```python
from build123d import *

# Parameters (mm, degrees)
BOSS_EXTRUDE1_DEPTH = 18
SKETCH2_R           = 12.45
SKETCH2_R_2         = 9.45
BOSS_EXTRUDE2_DEPTH = 10
SKETCH3_R           = 12.45
BOSS_EXTRUDE3_DEPTH = 2
CUT_EXTRUDE1_REACH  = 30.085
SKETCH4_R           = 1.45
CUT_EXTRUDE2_START  = -8
CUT_EXTRUDE2_DEPTH  = 3
CUT_EXTRUDE3_REACH  = 35.076
BOSS_EXTRUDE4_START = -5
BOSS_EXTRUDE4_DEPTH = 5
SKETCH8_R           = 1.5
CUT_EXTRUDE4_DEPTH  = 30.783714089


with BuildPart() as part:
    # Sketch1 → Boss-Extrude1 (new body)
    with BuildSketch(Plane(origin=(0, 0, 0), x_dir=(1, 0, 0), z_dir=(0, 1, 0))):
        with BuildLine():
            Line((-5.149418526, 2.325078245), (-5.149418526, -2.325078245))
            ThreePointArc((-5.149418526, -2.325078245), (5.65, 0), (-5.149418526, 2.325078245))
        make_face()
        with BuildLine():
            Line((-2.124418526, 1.541904967), (-2.124418526, -1.541904967))
            ThreePointArc((-2.124418526, -1.541904967), (2.625, 0), (-2.124418526, 1.541904967))
        make_face(mode=Mode.SUBTRACT)
    extrude(amount=BOSS_EXTRUDE1_DEPTH)



with BuildPart() as body_2:
    # Sketch2 → Boss-Extrude2 (new body)
    with BuildSketch(Plane.XZ):
        with Locations(Location((0, 0, 0), (0, 0, 270))):
            Circle(SKETCH2_R)
        with Locations(Location((0, 0, 0), (0, 0, 270))):
            Circle(SKETCH2_R_2, mode=Mode.SUBTRACT)
    extrude(amount=BOSS_EXTRUDE2_DEPTH)


with BuildPart() as part_1:
    add(part.part)

    add(body_2.part)  # Boss-Extrude3 merges body 2
    # Sketch3 → Boss-Extrude3 (add)
    with BuildSketch(Plane.XZ):
        with Locations(Location((0, 0, 0), (0, 0, 270))):
            Circle(SKETCH3_R)
    extrude(amount=BOSS_EXTRUDE3_DEPTH)

    # Sketch4 → Cut-Extrude1 (cut, up to next)
    with BuildSketch(Plane.ZY.offset(5.149418526), mode=Mode.PRIVATE) as cut_extrude1_sk1:
        with Locations((0, 14)):
            Circle(SKETCH4_R)
    cut_extrude1_tool1 = extrude(cut_extrude1_sk1.sketch, amount=-CUT_EXTRUDE1_REACH, mode=Mode.PRIVATE) & part_1.part
    # Sketch4 → Cut-Extrude1 (cut, up to next)
    with BuildSketch(Plane.ZY.offset(5.149418526), mode=Mode.PRIVATE) as cut_extrude1_sk2:
        with Locations((0, 4)):
            Circle(SKETCH4_R)
    cut_extrude1_tool2 = extrude(cut_extrude1_sk2.sketch, amount=-CUT_EXTRUDE1_REACH, mode=Mode.PRIVATE) & part_1.part
    add(cut_extrude1_tool1.solids().sort_by_distance((-5.149419, 14, 0))[0], mode=Mode.SUBTRACT)
    add(cut_extrude1_tool2.solids().sort_by_distance((-5.149419, 4, 0))[0], mode=Mode.SUBTRACT)

    # Sketch5 → Cut-Extrude2 (cut)
    with BuildSketch(Plane.XZ.offset(10).offset(CUT_EXTRUDE2_START)):
        with BuildLine():
            Line((-8.961166219, 3), (-12.083149424, 3))
            ThreePointArc((-12.083149424, 3), (0, 12.45), (12.083149424, 3))
            Line((12.083149424, 3), (8.961166219, 3))
            ThreePointArc((8.961166219, 3), (0, 9.45), (-8.961166219, 3))
        make_face()
        with BuildLine():
            Line((-8.961166219, -3), (-12.083149424, -3))
            ThreePointArc((-12.083149424, -3), (0, -12.45), (12.083149424, -3))
            Line((12.083149424, -3), (8.961166219, -3))
            ThreePointArc((8.961166219, -3), (0, -9.45), (-8.961166219, -3))
        make_face()
    extrude(amount=CUT_EXTRUDE2_DEPTH, mode=Mode.SUBTRACT)

    # Sketch6 → Cut-Extrude3 (cut, up to next)
    with BuildSketch(Plane.XZ.offset(10), mode=Mode.PRIVATE) as cut_extrude3_sk1:
        with BuildLine():
            Line((0.75, 9.420191081), (0.75, 12.427389106))
            ThreePointArc((0.75, 12.427389106), (0, 12.45), (-0.75, 12.427389106))
            Line((-0.75, 12.427389106), (-0.75, 9.420191081))
            ThreePointArc((-0.75, 9.420191081), (0, 9.45), (0.75, 9.420191081))
        make_face()
    cut_extrude3_tool1 = extrude(cut_extrude3_sk1.sketch, amount=-CUT_EXTRUDE3_REACH, mode=Mode.PRIVATE) & part_1.part
    # Sketch6 → Cut-Extrude3 (cut, up to next)
    with BuildSketch(Plane.XZ.offset(10), mode=Mode.PRIVATE) as cut_extrude3_sk2:
        with BuildLine():
            Line((0.75, -9.420191081), (0.75, -12.427389106))
            ThreePointArc((0.75, -12.427389106), (0, -12.45), (-0.75, -12.427389106))
            Line((-0.75, -12.427389106), (-0.75, -9.420191081))
            ThreePointArc((-0.75, -9.420191081), (0, -9.45), (0.75, -9.420191081))
        make_face()
    cut_extrude3_tool2 = extrude(cut_extrude3_sk2.sketch, amount=-CUT_EXTRUDE3_REACH, mode=Mode.PRIVATE) & part_1.part
    add(cut_extrude3_tool1.solids().sort_by_distance((0, -10, 10.941262))[0], mode=Mode.SUBTRACT)
    add(cut_extrude3_tool2.solids().sort_by_distance((0, -10, -10.941262))[0], mode=Mode.SUBTRACT)

    # Sketch7 → Boss-Extrude4 (add)
    with BuildSketch(Plane.XZ.offset(10).offset(BOSS_EXTRUDE4_START)):
        with BuildLine():
            ThreePointArc((-2.25, 12.244998979), (-1.502769623, 12.35897178), (-0.75, 12.427389106))
            Line((-0.75, 12.427389106), (-0.75, 18.627389106))
            Line((-0.75, 18.627389106), (-2.25, 18.627389106))
            Line((-2.25, 18.627389106), (-2.25, 12.244998979))
        make_face()
        with BuildLine():
            Line((2.25, 12.244998979), (2.25, 18.627389106))
            Line((2.25, 18.627389106), (0.75, 18.627389106))
            Line((0.75, 18.627389106), (0.75, 12.427389106))
            ThreePointArc((0.75, 12.427389106), (1.502769623, 12.35897178), (2.25, 12.244998979))
        make_face()
        with BuildLine():
            ThreePointArc((-0.75, -12.427389106), (-1.502769623, -12.35897178), (-2.25, -12.244998979))
            Line((-2.25, -12.244998979), (-2.25, -18.627389106))
            Line((-2.25, -18.627389106), (-0.75, -18.627389106))
            Line((-0.75, -18.627389106), (-0.75, -12.427389106))
        make_face()
        with BuildLine():
            Line((2.25, -18.627389106), (2.25, -12.244998979))
            ThreePointArc((2.25, -12.244998979), (1.502769623, -12.35897178), (0.75, -12.427389106))
            Line((0.75, -12.427389106), (0.75, -18.627389106))
            Line((0.75, -18.627389106), (2.25, -18.627389106))
        make_face()
    extrude(amount=BOSS_EXTRUDE4_DEPTH)

    # Sketch8 → Cut-Extrude4 (cut, through all)
    with BuildSketch(Plane.ZY.offset(2.25)):
        with Locations(Location((-15.436194043, -7.5, 0), (0, 0, 180))):
            Circle(SKETCH8_R)
        with Locations((15.436194043, -7.5)):
            Circle(SKETCH8_R)
    extrude(amount=-CUT_EXTRUDE4_DEPTH, mode=Mode.SUBTRACT)


solid = part_1.part
```
Part model, mm, in its own coordinate system. A direction names the side the tool comes from. Give positions to 0.01 mm unless a question says otherwise; leave off trailing zeros. Order: outer loops, then holes, each group sorted by start corner. A loop starts at its lowest first (then second) coordinate and runs counter-clockwise, first axis right, second up. Notation, with made-up numbers: M 14,74 L 39,74 A22 ccw 39,101 Z; hole C 37,-38 d6. An arc over 180 degrees is marked long. Use a Markdown table: item, result. Add a question column.
(1) Mould opens along Z. For faces 1 (the face through (1, -7, -18.627)), 2 (the face through (1.49, -6.925, -16.822)), 3 (the face through (-9.448, -6.833, 0.197)), 4 (the face through (2.25, -5.8, -15.5)) say: +Z half, -Z half, draft (parallel to the pull), parting line (faces both ways), or undercut.
(2) Saw through at A-A, the plane z = 0. Give the cut face in (x, y) (3 decimals).
(3) 3-axis set-ups, long thin cutter, end or side, ignore diameter. For faces 5 (the face through (2.25, -5.8, 15.4)), 6 (the face through (-2.124, 9, 0)), 7 (the face through (11, -3, -3)): which of +Z, -Z, +X, -X, +Y, -Y reach the whole face in a straight line?
(4) Saw through at B-B, the plane y = -7.5. Give the number of separate pieces and of enclosed holes in the cut face, and give its area (3 significant figures).
(5) Saw through at C-C, the plane x = -1.5. Give the cut face in (y, z).
(6) Saw through at D-D, the plane x = 7. Give the cut face in (y, z), and give its area (3 significant figures).
(7) Probe line 1 along Y through (x, z) = (-3.65, 0); line 2 along Y through (x, z) = (-9.25, 5.5); line 3 along Y through (x, z) = (-7, 4.5). List the from-to ranges inside material, lowest first. Write a range as [from, to].
(8) Drop flat-ended pins along their axis: P1, Ø10, axis at x = 8.5, y = -1, coming from the -Z side; P2, Ø8, axis at x = 8.5, z = -7, coming from the +Y side; P3, Ø2.5, axis at y = 11.5, z = -0.5, coming from the +X side. Give the stop position or say it passes through.
Answer key:
| question | item | result |
|---|---|---|
| 1 | face 1 | -Z half |
| 1 | face 2 | undercut |
| 1 | face 3 | undercut |
| 1 | face 4 | draft |
| 2 | outline | M -12.45,-10 L -9.45,-10 L -9.45,-2 L 9.45,-2 L 9.45,-10 L 12.45,-10 L 12.45,0 L 5.65,0 L 5.65,18 L 2.625,18 L 2.625,0 L -2.124,0 L -2.124,2.55 L -5.149,2.55 L -5.149,0 L -12.45,0 Z; M -5.149,5.45 L -2.124,5.45 L -2.124,12.55 L -5.149,12.55 Z; M -5.149,15.45 L -2.124,15.45 L -2.124,18 L -5.149,18 Z |
| 3 | face 5 | +Z, +X, +Y, -Y |
| 3 | face 6 | +Y |
| 3 | face 7 | -Z, +X, -X |
| 4 | separate pieces | 6 |
| 4 | enclosed holes | 0 |
| 4 | area | 217 mm^2 |
| 5 | outline | M -10,-18.63 L -5,-18.63 L -5,-9.33 L -10,-9.33 Z; M -10,9.33 L -5,9.33 L -5,18.63 L -10,18.63 Z; M -2,-12.36 L 0,-12.36 L 0,-5.45 L 18,-5.45 L 18,-2.15 L 0,-2.15 L 0,2.15 L 18,2.15 L 18,5.45 L 0,5.45 L 0,12.36 L -2,12.36 Z; hole C -7.5,-15.44 d3; hole C -7.5,15.44 d3 |
| 6 | outline | M -10,-10.3 L -5,-10.3 L -5,-6.35 L -10,-6.35 Z; M -10,6.35 L -5,6.35 L -5,10.3 L -10,10.3 Z; M -2,-10.3 L 0,-10.3 L 0,10.3 L -2,10.3 Z |
| 6 | area | 80.7 mm^2 |
| 7 | line 1 | [-2, 2.55], [5.45, 12.55], [15.45, 18] |
| 7 | line 2 | [-10, -5], [-2, 0] |
| 7 | line 3 | [-2, 0] |
| 8 | P1 | z = -11.95 |
| 8 | P2 | y = 0 |
| 8 | P3 | x = 5.65 |
